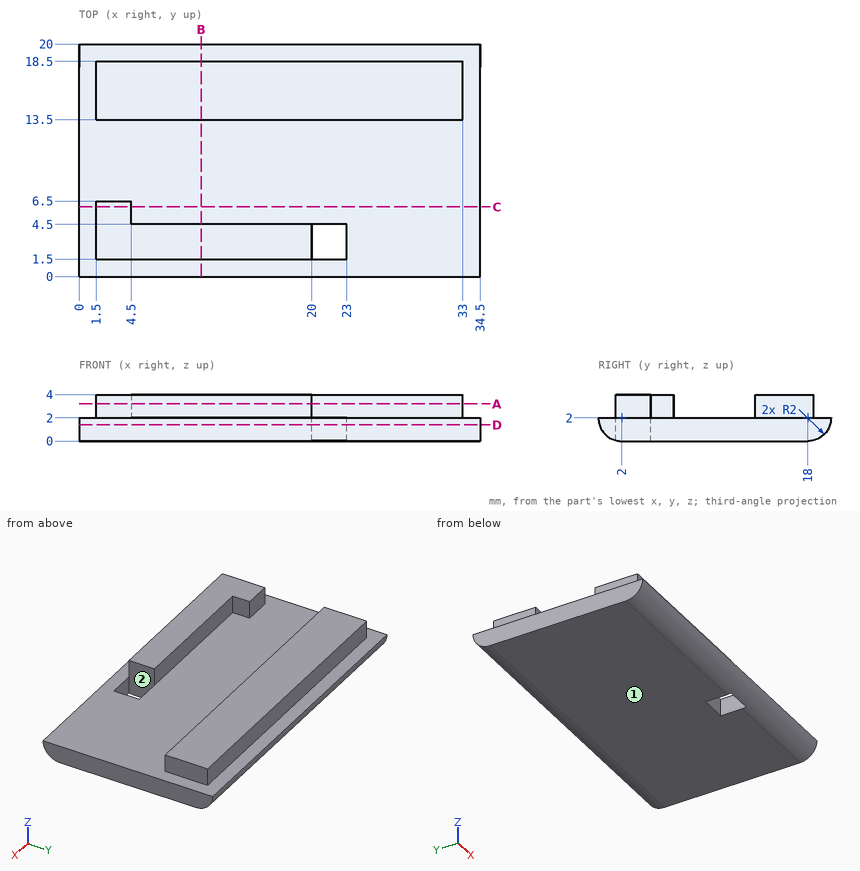
Print and shaded views of the part. All mm, measured from the part's lowest x, y and z. A direction names the side the tool comes from. Give positions to 0.01 mm unless a question says otherwise; leave off trailing zeros. Loops run counter-clockwise (first coordinate to the right, second up) from the corner with the lowest first, then second, coordinate; pieces in that order, holes last. Notation, with made-up numbers: M 72,14 L 113,14 A31 ccw 113,49 Z; hole C 61.25,35 d10. An arc over 180 degrees is marked long. Write each question's results on one line, items separated by ' | '.
Q1. Band-saw the part on C-C on y = 6. Write the cut outline in (x, z), and give its area (3 significant figures).
Geometry check:
outline: M 0,0 L 34.5,0 L 34.5,2 L 4.5,2 L 4.5,4 L 1.5,4 L 1.5,2 L 0,2 Z | area: 75.0 mm²
Q2. Which spindle directions (+Z, -Z, +X, -X, +Y, -Y) get a long thin tool onto all of the face, cutting with end or side? Do the marked faces 1 and 2. Say none if no direction does.
Geometry check:
face 1: -Z, +X, -X, +Y, -Y | face 2: +Z, -Z
Q3. Band-saw the part on A-A on z = 3.2. Write the cut outline in (x, y).
Geometry check:
outline: M 1.5,1.5 L 20,1.5 L 20,4.5 L 4.5,4.5 L 4.5,6.5 L 1.5,6.5 Z; M 1.5,13.5 L 33,13.5 L 33,18.5 L 1.5,18.5 Z
Q4. Band-saw the part on B-B on x = 10.5. Write the cut outline in (y, z).
Geometry check:
outline: M 0,2 A2 ccw 2,0 L 18,0 A2 ccw 20,2 L 18.5,2 L 18.5,4 L 13.5,4 L 13.5,2 L 4.5,2 L 4.5,4 L 1.5,4 L 1.5,2 Z
Q5. Probe probe 1 along Y at (x, z) = (9.5, 2.75); probe 2 along Z at (x, y) = (23, 12.5); probe 3 along Y at (x, z) = (2, 2.4). List the from-to ranges inside material, lowest first.
Geometry check:
probe 1: y = 1.5 to 4.5, 13.5 to 18.5 | probe 2: z = 0 to 2 | probe 3: y = 1.5 to 6.5, 13.5 to 18.5
Q6. Band-saw the part on D-D on z = 1.4. Write the cut outline in (x, y).
Geometry check:
outline: M 0,0.09 L 34.5,0.09 L 34.5,19.91 L 0,19.91 Z; hole M 20,1.5 L 23,1.5 L 23,4.5 L 20,4.5 Z
Q7. Flat gauge pins, fed straight in: P1, Ø0.6, axis at x = 21.5, z = 1, coming from the +Y side; P2, Ø1.5, axis at y = 3, z = 2.5, coming from the +X side; P3, Ø1, axis at x = 2.5, z = 3, coming from the +Y side; P4, Ø4, axis at x = 6.5, y = 10, coming from the +Z side. Where does each tip first touch, or does it go through?
Geometry check:
P1: stops at y = 19.87 | P2: stops at x = 34.5 | P3: stops at y = 18.5 | P4: stops at z = 2
